Check sheet for the modelled part. Datum: model origin and axes. Units: mm. Face numbers are marked on the shaded views. Give positions to 0.01 mm unless a question says otherwise; leave off trailing zeros. Order: outer loops, then holes, each group sorted by start corner. A loop starts at its lowest first (then second) coordinate and runs counter-clockwise, first axis right, second up.
Item 1: Sectioned sample at C-C on x = -5. Record the boundary of the cut face in (y, z) (3 decimals), and give its area (3 significant figures).
Item 2: Material ranges on line 1 along Z through (x, y) = (-11.5, 0); line 2 along Y through (x, z) = (-13, 6) (3 decimals); line 3 along Y through (x, z) = (0, 7) (3 decimals), recorded low to high.
Item 3: Gauge pin test, flat ends, axial feed: P1, Ø0.6, axis at x = 8, z = 13, coming from the +Y side; P2, Ø1.5, axis at y = -6, z = 4.5, coming from the +X side; P3, Ø2, axis at y = 8, z = 15, coming from the +X side. Record the tip position at first contact, or that the pin passes through.
Item 4: Sectioned sample at A-A on y = 0. Record the boundary of the cut face in (x, z) (3 decimals), and give its area (3 significant figures).
Item 5: Sectioned sample at D-D on z = 22.25. Record the boundary of the cut face in (x, y) (3 decimals), and give its area (3 significant figures).
Item 6: Sectioned sample at B-B on z = 19. Record the boundary of the cut face in (x, y) (3 decimals), and give its area (3 significant figures).
Item 7: Release check for a two-part mould opening along Y. For the marked faces 1, 2, 3 and 4 record: released by +Y, released by -Y, zero draft, split by the parting line, or undercut.
Autodesk Fusion 360 part; units mm, degrees
sketch "Sketch1" plane through (0, 0, 0) normal (0, 0, 1) x (1, 0, 0)
  line L0 (17.5, 3) -> (-7.01, 3)
  line L1 (17.5, -3) -> (17.5, 3)
  arc A0 (7.01, 3) -> (7.01, -3) centre (0, 0) ccw
  arc A1 (10.1927, 3) -> (10.1927, -3) centre (0, 0) ccw
  line L2 (-7.01, -3) -> (17.5, -3)
  dimension "d1" = 15.25
extrude "Extrude1" add sketch "Sketch1" along normal blind 25 contours L0 A0 A1 L2 makes body 1
sketch "Sketch3" plane through (0, 0, 0) normal (0, 0, 1) x (1, 0, 0)
  arc A0 (7.01, 3) -> (7.01, -3) centre (0, 0) ccw construction
  line L0 (0, -10.625) -> (-15.125, -10.625)
  line L1 (-15.125, -10.625) -> (-15.125, 10.625)
  line L2 (-15.125, 10.625) -> (0, 10.625)
  arc A1 (10.1927, 3) -> (10.1927, -3) centre (0, 0) ccw
  line L3 (0, 10.625) -> (0, 7.625)
  line L4 (0, -7.625) -> (0, -10.625)
extrude "Extrude2" add sketch "Sketch3" along normal blind 25 bodies 1
ref_plane "WorkPlane1" through (-12.125, 0, 12.5) normal (-1, 0, 0) x (0, -1, 0)
sketch "Sketch4" plane through (-15.125, 0, 0) normal (-1, 0, 0) x (0, -1, 0)
  line L0 (-10.625, 0) -> (10.625, 0)
  line L1 (10.625, 0) -> (10.625, 25)
  line L2 (10.625, 25) -> (-10.625, 25)
  line L3 (-10.625, 25) -> (-10.625, 0)
  line L4 (0, 25) -> (0, 19) construction
  line L5 (0, 0) -> (0, 6) construction
  dimension "d11" = 6
  dimension "d12" = 6
hole "Hole1" at (-15.125, 0, 19) direction (1, 0, 0) diameter 3 end through all bodies 1 1
hole "Hole2" at (-15.125, 0, 6) direction (1, 0, 0) diameter 3 depth 24.216 tip angle 180 bodies 1
ref_plane "WorkPlane2" through (-5.125, 0, 12.5) normal (-1, 0, 0) x (0, -1, 0)
sketch "Sketch5" plane through (-5.125, 0, 12.5) normal (-1, 0, 0) x (0, 1, 0)
  line L0 (7.625, -12.5) -> (-7.625, -12.5) construction
  line L1 (0, -12.5) -> (0, -6.5) construction
  line L2 (-10.625, 12.5) -> (10.625, 12.5) construction
  line L3 (0, 12.5) -> (0, 6.5) construction
  point P0 (0, -12.5)
  point P1 (0, 12.5)
  dimension "d20" = 6
  dimension "d21" = 6
hole "Hole3" at (-5.125, 0, 19) direction (1, 0, 0) diameter 6 depth 7 tip angle 180 bodies 1
hole "Hole4" at (-5.125, 0, 6) direction (1, 0, 0) diameter 6 depth 7 tip angle 180 bodies 1
fillet "Fillet1" radius 1 4 edges at (10.1927, -3, 12.5) (7.01, -3, 12.5) (10.1927, 3, 12.5) (7.01, 3, 12.5) on bodies 1
copy_body "Body->Comp1" bodies 1 removing the originals makes body 2 in component "Mountable Linear Bearing Holder"
component "Mountable Linear Bearing Holder" placed x (1, 0, 0) y (0, 1, 0) z (0, 0, 1) at (0, 0, 0)
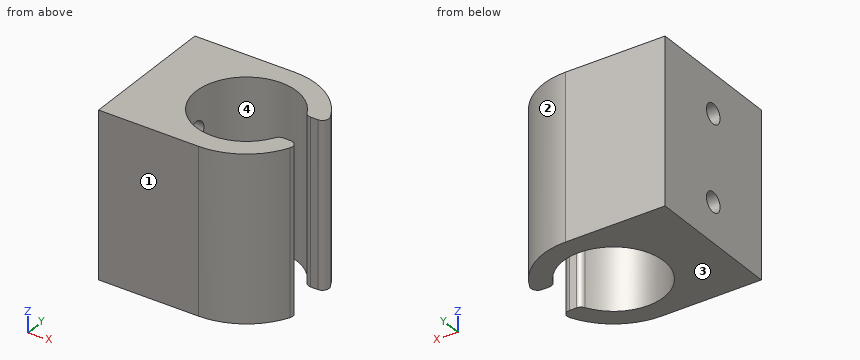
Report:
1. outline: (-10.625, 0) - (-5.757, 0) - (-5.757, 25) - (-10.625, 25) - close; (5.757, 0) - (10.625, 0) - (10.625, 25) - (5.757, 25) - close
1. area: 243 mm2
2. line 1: z = 0 to 4.5, 7.5 to 17.5, 20.5 to 25
2. line 2: y = -10.625 to -1.5, 1.5 to 10.625
2. line 3: y = -10.625 to -7.625, 7.625 to 10.625
3. P1: stops at y = 7.32
3. P2: stops at x = 9.24
3. P3: stops at x = 7.99
4. outline: (-15.125, 0) - (-7.625, 0) - (-7.625, 4.5) - (-15.125, 4.5) - close; (-15.125, 7.5) - (-7.625, 7.5) - (-7.625, 17.5) - (-15.125, 17.5) - close; (-15.125, 20.5) - (-7.625, 20.5) - (-7.625, 25) - (-15.125, 25) - close
4. area: 143 mm2
5. outline: (-15.125, -10.625) - (0, -10.625) arc R10.625 ccw to (9.664, -4.416) arc R1 ccw to (8.754, -3) - (7.641, -3) arc R1 ccw to (6.755, -3.536) arc R7.625 cw (long way) to (6.755, 3.536) arc R1 ccw to (7.641, 3) - (8.754, 3) arc R1 ccw to (9.664, 4.416) arc R10.625 ccw to (0, 10.625) - (-15.125, 10.625) - close
5. area: 297 mm2
6. outline: (-15.125, -10.625) - (0, -10.625) arc R10.625 ccw to (9.664, -4.416) arc R1 ccw to (8.754, -3) - (7.641, -3) arc R1 ccw to (6.755, -3.536) arc R7.625 cw to (-7.476, -1.5) - (-15.125, -1.5) - close; (-15.125, 1.5) - (-7.476, 1.5) arc R7.625 cw to (6.755, 3.536) arc R1 ccw to (7.641, 3) - (8.754, 3) arc R1 ccw to (9.664, 4.416) arc R10.625 ccw to (0, 10.625) - (-15.125, 10.625) - close
6. area: 274 mm2
7. face 1: released by -Y
7. face 2: released by +Y
7. face 3: zero draft
7. face 4: undercut
